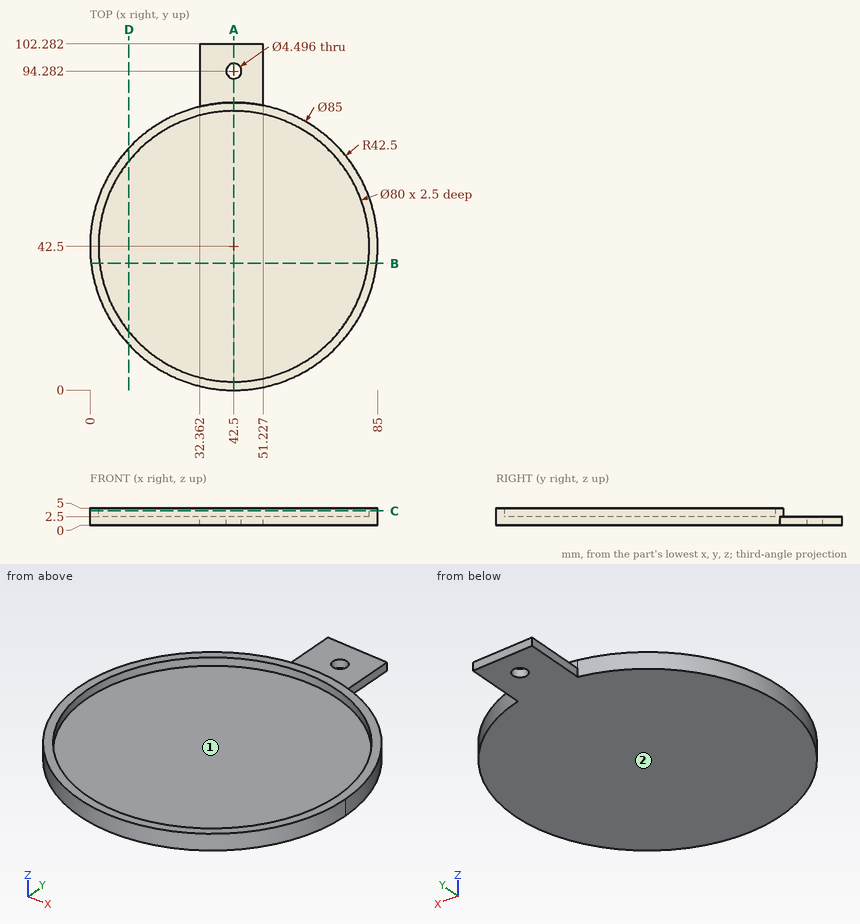
Geometry: see drawing. Coordinates: mm, zero at the bounding-box minimum. Give positions to 0.01 mm unless a question says otherwise; leave off trailing zeros. Order: outer loops, then holes, each group sorted by start corner. A loop starts at its lowest first (then second) coordinate and runs counter-clockwise, first axis right, second up. Notation, with made-up numbers: (55, 79) - (111, 79) arc R14 ccw to (111, 88) - close; hole circle Ø5 at (76.5, 13.5). An arc over 180 degrees is marked (long way). One line per item, written item: value.
1. Cut plane B-B, the plane y = 37.5. Output: boundary loops of the cut face in (x, z) (1 decimal).
Determined:
outline: (0.3, 0) - (84.7, 0) - (84.7, 5) - (82.2, 5) - (82.2, 2.5) - (2.8, 2.5) - (2.8, 5) - (0.3, 5) - close
2. Line query: probe 1 along Y at (x, z) = (42.5, 1.15); probe 2 along Y at (x, z) = (42.5, 4.45). Output: solid intervals per line, ascending.
Determined:
probe 1: 0 to 92.03, 96.53 to 102.28
probe 2: 0 to 2.5, 82.5 to 85
3. Pin query (flat end, axial travel): pin 1 Ø24 at (x, y) = (29.5, 36) entering from +Z; pin 2 Ø2 at (y, z) = (96.5, 1.5) entering from +X; pin 3 Ø20.5 at (x, y) = (45, 90.5) entering from +Z; pin 4 Ø1.2 at (y, z) = (93, 2) entering from -X. Return the tip coordinate at first contact, or that it passes through.
Determined:
pin 1: z = 2.5
pin 2: x = 51.23
pin 3: z = 5
pin 4: x = 32.36
4. Cut plane C-C, the plane z = 4.25. Output: boundary loops of the cut face in (x, y).
Determined:
outline: circle Ø85 at (42.5, 42.5); hole circle Ø80 at (42.5, 42.5)
5. Cut plane A-A, the plane x = 42.5. Output: boundary loops of the cut face in (y, z), and give its area (3 significant figures).
Determined:
outline: (0, 0) - (92.03, 0) - (92.03, 2.5) - (85, 2.5) - (85, 5) - (82.5, 5) - (82.5, 2.5) - (2.5, 2.5) - (2.5, 5) - (0, 5) - close; (96.53, 0) - (102.28, 0) - (102.28, 2.5) - (96.53, 2.5) - close
area: 257 mm2
6. Cut plane D-D, the plane x = 11.5. Output: boundary loops of the cut face in (y, z).
Determined:
outline: (13.43, 0) - (71.57, 0) - (71.57, 5) - (67.78, 5) - (67.78, 2.5) - (17.22, 2.5) - (17.22, 5) - (13.43, 5) - close
7. Draft query along Y for the marked faces 1 and 2. Return one class per face: released by +Y, released by -Y, zero draft, split by the parting line, or undercut.
Determined:
face 1: undercut
face 2: zero draft
